Drawing for the job (mm, zero at the part's lowest x, y, z). A direction names the side the tool comes from. Coordinates: 2 decimals unless noted, no trailing zeros. Loops run counter-clockwise (first coordinate to the right, second up) from the corner with the lowest first, then second, coordinate; pieces in that order, holes last.
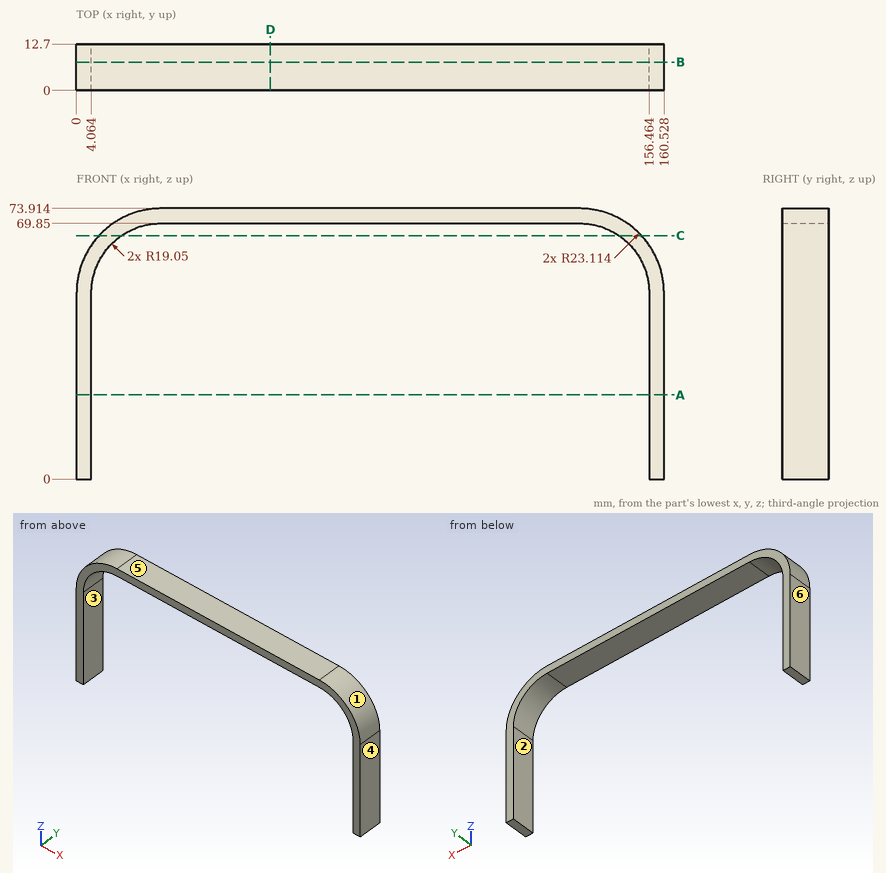
Q1. Saw through at C-C (z = 66.5). List the corners of the cut face in (x, y), plus the area to 3 significant figures.
Q2. Probe line 1 (X direction, y = 7.5, z = 21.5); line 2 (Z direction, x = 101.5, y = 2); line 3 (X direction, y = 4.75, z = 53.5). List the from-to ranges inside material, lowest first.
Q3. Saw through at A-A (z = 23). List the corners of the cut face in (x, y), plus the area to 3 significant figures.
Q4. Mould opens along X. For the marked faces 3, 4, 5 and 6 say: released by +X, released by -X, zero draft, split by the parting line, or undercut.
Q5. Saw through at D-D (x = 53). List the corners of the cut face in (y, z), plus the area to 3 significant figures.
Q6. Tool access for the marked faces 1 and 2: list every direction of +Z, -Z, +X, -X, +Y, -Y with a clear straight run to the whole face (end or side of a thin tool).
Q7. Drop flat-ended pins along their axis: P1, Ø5, axis at y = 5.5, z = 34.5, coming from the -X side; P2, Ø1.5, axis at y = 2, z = 54, coming from the -X side. Give the stop position or say it passes through.
Q8. Saw through at B-B (y = 7.75). List the corners of the cut face in (x, z), plus the area to 3 significant figures.
Checked values:
1. outline: (6.15, 0) - (12.32, 0) - (12.32, 12.7) - (6.15, 12.7) - close; (148.2, 0) - (154.38, 0) - (154.38, 12.7) - (148.2, 12.7) - close
1. area: 157 mm2
2. line 1: x = 0 to 4.06, 156.46 to 160.53
2. line 2: z = 69.85 to 73.91
2. line 3: x = 0.16 to 4.26, 156.27 to 160.37
3. outline: (0, 0) - (4.06, 0) - (4.06, 12.7) - (0, 12.7) - close; (156.46, 0) - (160.53, 0) - (160.53, 12.7) - (156.46, 12.7) - close
3. area: 103 mm2
4. face 3: undercut
4. face 4: released by +X
4. face 5: zero draft
4. face 6: released by -X
5. outline: (0, 69.85) - (12.7, 69.85) - (12.7, 73.91) - (0, 73.91) - close
5. area: 51.6 mm2
6. face 1: +Z, +X, +Y, -Y
6. face 2: -Z, +Y, -Y
7. P1: stops at x = 0
7. P2: stops at x = 0.13
8. outline: (0, 0) - (4.06, 0) - (4.06, 50.8) arc R19.05 cw to (23.11, 69.85) - (137.41, 69.85) arc R19.05 cw to (156.46, 50.8) - (156.46, 0) - (160.53, 0) - (160.53, 50.8) arc R23.11 ccw to (137.41, 73.91) - (23.11, 73.91) arc R23.11 ccw to (0, 50.8) - close
8. area: 1,150 mm2
